Source: CAD feature listing. Evaluate the final solid. Frame: model axes, mm. Give positions to 0.01 mm unless a question says otherwise; leave off trailing zeros. Order: outer loops, then holes, each group sorted by start corner. A loop starts at its lowest first (then second) coordinate and runs counter-clockwise, first axis right, second up. Notation, with made-up numbers: (13, 48) -> (64, 48) arc R31 cw to (64, 76) -> close; hole circle Ø7 at (9.25, 87.25). An arc over 180 degrees is marked (long way). Answer in a Markdown table with one row per item.
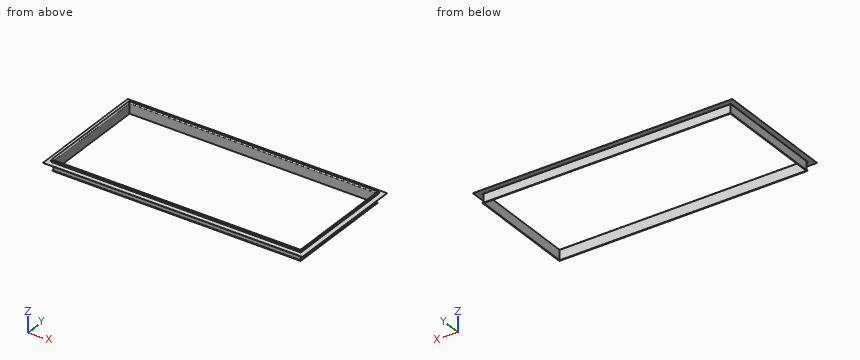
```python
from build123d import *


with BuildPart() as f2:
    # F2: sweep along a path in F1
    with BuildLine(Plane.XY) as f2_path:
        Line((0, 6), (1663.7, 6))
        Line((1663.7, 6), (1663.7, -736.95))
        Line((1663.7, -736.95), (0, -736.95))
        Line((0, -736.95), (0, 6))
    # F0 (on Right) → F2 (sweep)
    with BuildSketch(Plane.YZ):
        with BuildLine():
            Line((0, -6), (0, -70.7))
            Line((0, -70.7), (6, -70.7))
            Line((6, -70.7), (6, -68))
            Line((6, -68), (4.8, -68))
            Line((4.8, -68), (4.8, -69.5))
            Line((4.8, -69.5), (1.5, -69.5))
            Line((1.5, -69.5), (1.5, -6))
            ThreePointArc((1.5, -6), (2.8180194847, -2.8180194847), (6, -1.5))
            Line((6, -1.5), (8.6, -1.5))
            Line((8.6, -1.5), (8.6, -9.4503759398))
            Line((8.6, -9.4503759398), (6, -12.5))
            Line((6, -12.5), (6, -13.7))
            Line((6, -13.7), (6.5538461538, -13.7))
            Line((6.5538461538, -13.7), (8.6, -11.3))
            Line((8.6, -11.3), (8.6, -13.7))
            Line((8.6, -13.7), (43.1, -13.7))
            Line((43.1, -13.7), (43.1, -12.5))
            Line((43.1, -12.5), (9.8, -12.5))
            Line((9.8, -12.5), (9.8, -4.5))
            Line((9.8, -4.5), (13.5, -4.5))
            Line((13.5, -4.5), (13.5, -3.3))
            Line((13.5, -3.3), (9.8, -3.3))
            Line((9.8, -3.3), (9.8, -1.5))
            Line((9.8, -1.5), (12.2, -1.5))
            Line((12.2, -1.5), (12.2, 0))
            Line((12.2, 0), (6, 0))
            ThreePointArc((6, 0), (1.7573593129, -1.7573593129), (0, -6))
        make_face()
    sweep(path=f2_path.line, transition=Transition.RIGHT)


solid = f2.part
```
(1) First-contact query: pin 1 Ø10 at (y, z) = (-454.5, -57) entering from +X; pin 2 Ø1.2 at (y, z) = (-392.5, -69) entering from -X; pin 3 Ø1.4 at (x, z) = (775, -2.5) entering from -Y. Flat tips, straight axial feed; report the tip coordinate or a pass-through.
A:
| item | result |
|---|---|
| pin 1 | stops at x = 1659.2 |
| pin 2 | stops at x = 0 |
| pin 3 | stops at y = -740.75 |
(2) Section query A-A (z = -29). Return the cut outline in (x, y).
A:
| item | result |
|---|---|
| outline | (4.5, -732.45) -> (1659.2, -732.45) -> (1659.2, 1.5) -> (4.5, 1.5) -> close; hole (6, -730.95) -> (1657.7, -730.95) -> (1657.7, 0) -> (6, 0) -> close |
(3) Ray query, probe 1 along Y at (x, z) = (1469.5, -5.5); probe 2 along Y at (x, z) = (385.5, -65.5); probe 3 along X at (y, z) = (-12, -28). Return the intervals inside material, ascending.
A:
| item | result |
|---|---|
| probe 1 | y = -740.75 to -739.55, -732.48 to -730.97, 0.02 to 1.53, 8.6 to 9.8 |
| probe 2 | y = -732.45 to -730.95, 0 to 1.5 |
| probe 3 | x = 4.5 to 6, 1657.7 to 1659.2 |
